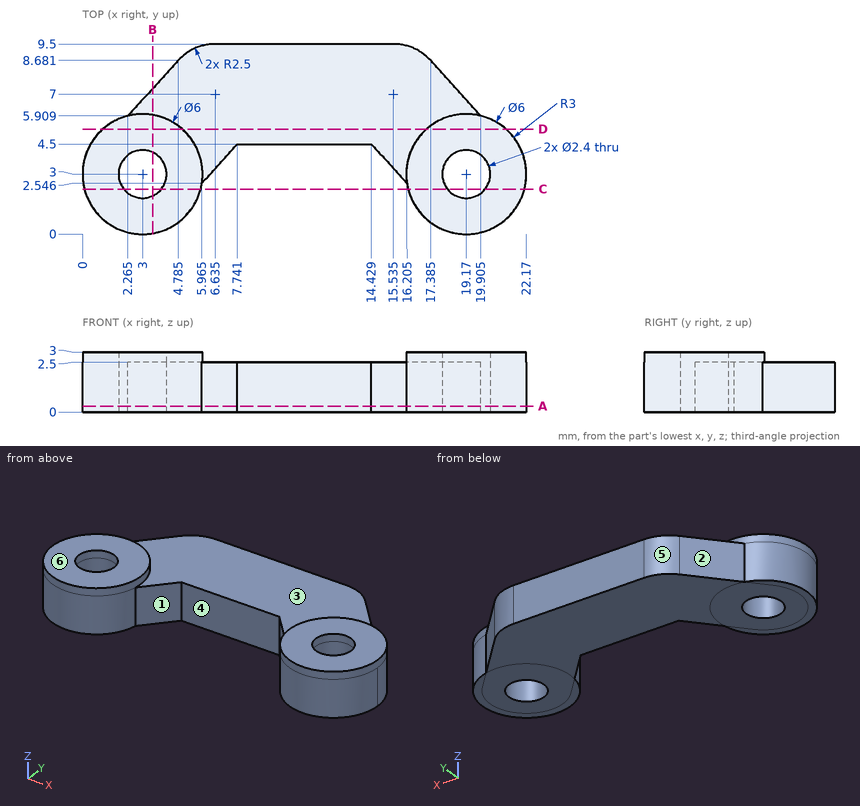
Can you work these out from the drawing? Everything is in mm from the part's minimum corner. A direction names the side the tool comes from. Round coordinates to 2 decimals unless told otherwise and drop trailing zeros. Order: outer loops, then holes, each group sorted by start corner. A loop starts at its lowest first (then second) coordinate and runs counter-clockwise, first axis right, second up. Notation, with made-up numbers: (60.25, 47.5) -> (116.25, 47.5) arc R22 ccw to (116.25, 71.5) -> close; hole circle Ø9 at (78.5, -29). An arc over 180 degrees is marked (long way). Return JSON: item names as keys, results as strings. Group by question number.
1. If we section it at D-D, the plane y = 5.25: Write out the boundary of the cut face in (x, z) (1 decimal).
2. Which directions (+Z, -Z, +X, -X, +Y, -Y) give clear straight access to the entire face, cutting with the end or side of a thin tool? Please do the marked faces 1, 2 and 3.
3. Will these pins go through, and if not, where does the flat tip stop? pin 1 (1.4 mm diameter, centred on x = 3, y = 3, fed in from +Z) (3 decimals); pin 2 (5.5 mm diameter, centred on x = 8, y = 6, fed in from +Z).
4. If we section it at B-B, the plane x = 3.5: Write out the boundary of the cut face in (y, z).
5. I need wall thicknesses on line 1 (X direction, y = 4, z = 1.25) (1 decimal); line 2 (Y direction, x = 3, z = 2.8); line 3 (Z direction, x = 14, y = 8.5). Which ranges of each line are inside material? Lowest first, please. Write a range as [from, to].
6. We'd pull the mould along X, two halves only. Please class the marked faces 4, 5 and 6: released by +X, released by -X, zero draft, split by the parting line, or undercut.
7. If we section it at C-C, the plane y = 2.25: Write out the boundary of the cut face in (x, z) (1 decimal).
8. If we section it at A-A, the plane z = 0.3: Write out the boundary of the cut face in (x, y) (1 decimal), then the cut area to 3 significant figures.
Output values:
{
 "1": {"outline": "(1, 0) -> (21.2, 0) -> (21.2, 3) -> (17.2, 3) -> (17.2, 2.5) -> (5, 2.5) -> (5, 3) -> (1, 3) -> close"},
 "2": {"face 1": "+Z, -Z, -Y", "face 2": "+Z, -Z, -X, +Y", "face 3": "+Z, +Y"},
 "3": {"pin 1": "through", "pin 2": "z = 2.5"},
 "4": {"outline": "(0.04, 0) -> (1.91, 0) -> (1.91, 3) -> (0.04, 3) -> close; (4.09, 0) -> (7.27, 0) -> (7.27, 2.5) -> (5.96, 2.5) -> (5.96, 3) -> (4.09, 3) -> close"},
 "5": {"line 1": "[0.2, 2.3], [3.7, 7.3], [14.9, 18.5], [19.8, 22]", "line 2": "[0, 1.8], [4.2, 6]", "line 3": "[0, 2.5]"},
 "6": {"face 4": "undercut", "face 5": "released by -X", "face 6": "zero draft"},
 "7": {"outline": "(0.1, 0) -> (2.1, 0) -> (2.1, 3) -> (0.1, 3) -> close; (3.9, 0) -> (5.9, 0) -> (5.9, 3) -> (3.9, 3) -> close; (16.3, 0) -> (18.2, 0) -> (18.2, 3) -> (16.3, 3) -> close; (20.1, 0) -> (22.1, 0) -> (22.1, 3) -> (20.1, 3) -> close"},
 "8": {"outline": "(2.3, 5.9) arc R3 ccw (long way) to (6, 2.5) -> (7.7, 4.5) -> (14.4, 4.5) -> (16.2, 2.5) arc R3 ccw (long way) to (19.9, 5.9) -> (17.4, 8.7) arc R2.5 ccw to (15.5, 9.5) -> (6.6, 9.5) arc R2.5 ccw to (4.8, 8.7) -> close; hole circle Ø2.4 at (3, 3); hole circle Ø2.4 at (19.2, 3)", "area": "120 mm²"}
}
